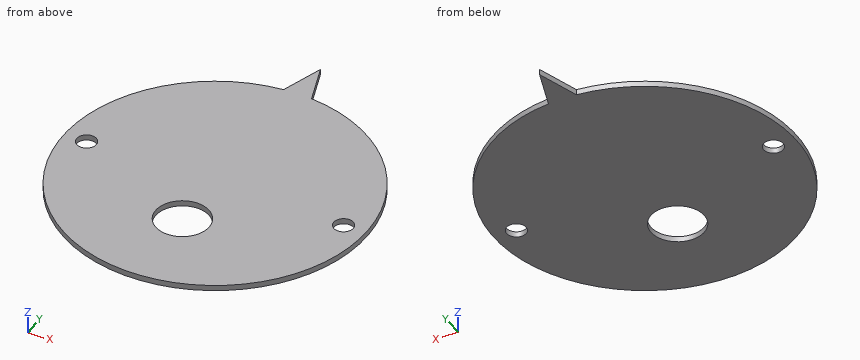
from build123d import *

# Parameters (mm, degrees)
F0_R       = 1.75
F0_R_2     = 4.75
F1_DEPTH   = 1
F2_SIZE2   = 2.5
F2_SIZE    = 7.465
F2_2_SIZE2 = 2.49999
F2_2_SIZE  = 7.46499


# Not quite as in the source:
# - a fillet or chamfer is up to 0.001 mm smaller than in the source, because OpenCascade refuses the exact size


with BuildPart() as f1:
    # F0 (on Top) → F1 (new body)
    with BuildSketch(Plane.XY):
        with BuildLine():
            Line((-2.5, 34.35), (-2.5, 26.8840101175))
            ThreePointArc((-2.5, 26.8840101175), (0, -27), (2.5, 26.8840101175))
            Line((2.5, 26.8840101175), (2.5, 34.35))
            Line((2.5, 34.35), (-2.5, 34.35))
        make_face()
        with Locations((-23, 0)):
            Circle(F0_R, mode=Mode.SUBTRACT)
        with Locations((0, -10.65)):
            Circle(F0_R_2, mode=Mode.SUBTRACT)
        with Locations((23, 0)):
            Circle(F0_R, mode=Mode.SUBTRACT)
    extrude(amount=F1_DEPTH)

    # F2
    f2_edges = [f1.edges().sort_by_distance(p)[0] for p in [
        (-2.5, 34.35, 0.5),
    ]]
    f2_side = f1.faces().sort_by_distance((-2.5, 30.617005, 0.5))[0]
    chamfer(f2_edges, length=F2_SIZE, length2=F2_SIZE2, reference=f2_side)

    # F2#2 (size 7.465 and 2.5 in the source; OpenCascade refuses exactly that, so slightly less here)
    f2_2_edges = [f1.edges().sort_by_distance(p)[0] for p in [
        (2.5, 34.35, 0.5),
    ]]
    f2_2_side = f1.faces().sort_by_distance((2.5, 30.617005, 0.5))[0]
    chamfer(f2_2_edges, length=F2_2_SIZE, length2=F2_2_SIZE2, reference=f2_2_side)


solid = f1.part
Work out the finished part from the listing and answer in its coordinate system (mm). Give positions to 0.01 mm unless a question says otherwise; leave off trailing zeros. Order: outer loops, then holes, each group sorted by start corner. A loop starts at its lowest first (then second) coordinate and runs counter-clockwise, first axis right, second up. Notation, with made-up numbers: M 68,71 L 112,71 A13 ccw 112,89 Z; hole C -20,8 d8. An arc over 180 degrees is marked long. Return JSON: item names as keys, results as strings.
Q1. Find section C-C, the plane y = -9.5. Write down the section's boundary in (x, z), and give its area (3 significant figures).
Answer below:
{"outline": "M -25.27,0 L -4.61,0 L -4.61,1 L -25.27,1 Z; M 4.61,0 L 25.27,0 L 25.27,1 L 4.61,1 Z", "area": "41.3 mm^2"}
Q2. Find section D-D, the plane x = 23. Write down the section's boundary in (y, z), and give its area (3 significant figures).
Answer below:
{"outline": "M -14.14,0 L -1.75,0 L -1.75,1 L -14.14,1 Z; M 1.75,0 L 14.14,0 L 14.14,1 L 1.75,1 Z", "area": "24.8 mm^2"}
Q3. Find the intervals of material crossed by line 1 along Y through (x, z) = (-23, 0.4); line 2 along Y through (x, z) = (-3, 0.6); line 3 along Y through (x, z) = (6, 0.5), in increasing order. Write a range as [from, to].
Answer below:
{"line 1": "y = [-14.14, -1.75], [1.75, 14.14]", "line 2": "y = [-26.83, -14.33], [-6.97, 26.83]", "line 3": "y = [-26.32, 26.32]"}
Q4. Find section B-B, the plane z = 0.4. State how many separate pieces and enclosed holes the cut face has, and give its area (3 significant figures).
Answer below:
{"separate pieces": "1", "enclosed holes": "3", "area": "2,220 mm^2"}
Q5. This flat-tipped pin is pushed along its axis until it touches: pin 1 (2 mm diameter, centred on x = -23, y = 0, fed in from -Z). Where does it stop, or does it pass through?
Answer below:
{"pin 1": "passes through"}
Q6. Find section A-A, the plane y = 0. Write down the section's boundary in (x, z).
Answer below:
{"outline": "M -27,0 L -24.75,0 L -24.75,1 L -27,1 Z; M -21.25,0 L 21.25,0 L 21.25,1 L -21.25,1 Z; M 24.75,0 L 27,0 L 27,1 L 24.75,1 Z"}
